Geometry: final body of the model. Coordinates: model frame, mm. Face numbers are marked on the shaded views. Round coordinates to 2 decimals unless told otherwise and drop trailing zeros. Loops run counter-clockwise (first coordinate to the right, second up) from the corner with the lowest first, then second, coordinate; pieces in that order, holes last. Notation, with made-up numbers: M 61,-37.5 L 100,-37.5 A21 ccw 100,-6.5 Z; hole C -16,67 d4. An arc over 180 degrees is marked long. Answer as a JSON object with one key per item and string values.
from build123d import *

# Parameters (mm, degrees)
SKETCH_1_W           = 300
SKETCH_1_H           = 30
EXTRUDE_1_DEPTH      = 20
EXTRUDE_2_DEPTH      = 28
EXTRUDE_2_DEPTH_BACK = 328
SKETCH_3_R           = 13.5
SKETCH_3_R_2         = 6
SKETCH_3_R_3         = 4
CUT_EXTRUDE_2_DEPTH  = 182.614977356
SKETCH_3_4_R         = 2.4
CUT_EXTRUDE_3_DEPTH  = 4.5
SKETCH_3_5_R         = 2.4
CUT_EXTRUDE_4_DEPTH  = 5


with BuildPart() as part:
    # Sketch 1 → Extrude 1 (new body)
    with BuildSketch(Plane.XY):
        with Locations((0, 15)):
            Rectangle(SKETCH_1_W, SKETCH_1_H)
    extrude(amount=EXTRUDE_1_DEPTH)

    # Sketch 2 → Extrude 2 (add, two sides: drawn at the far end of the back side and taken through both)
    with BuildSketch(Plane.ZY.offset(150).offset(-EXTRUDE_2_DEPTH_BACK)):
        with BuildLine():
            Line((0, 20), (0, 10))
            ThreePointArc((0, 10), (5, 15), (0, 20))
        make_face()
    extrude(amount=EXTRUDE_2_DEPTH + EXTRUDE_2_DEPTH_BACK)

    # Sketch 3 → Cut-Extrude 2 (cut, through all)
    # profile 1 of 3: a face of its own
    with BuildSketch(Plane(origin=(0, 0, 0), x_dir=(-1, 0, 0), z_dir=(0, 0, -1))):
        with Locations((0, 15)):
            Circle(SKETCH_3_R)
        with Locations((0, 15)):
            Circle(SKETCH_3_R_2, mode=Mode.SUBTRACT)
    # profile 2 of 3: a face of its own
    with BuildSketch(Plane(origin=(0, 0, 0), x_dir=(-1, 0, 0), z_dir=(0, 0, -1))):
        with Locations((0, 15)):
            Circle(SKETCH_3_R_2)
        with Locations((0, 15)):
            Circle(SKETCH_3_R_3, mode=Mode.SUBTRACT)
    # profile 3 of 3: a face of its own
    with BuildSketch(Plane(origin=(0, 0, 0), x_dir=(-1, 0, 0), z_dir=(0, 0, -1))):
        with Locations((0, 15)):
            Circle(SKETCH_3_R_3)
    extrude(amount=-CUT_EXTRUDE_2_DEPTH, mode=Mode.SUBTRACT)

    # Sketch 3_4 → Cut-Extrude 3 (cut)
    # profile 1 of 2: a face of its own
    with BuildSketch(Plane(origin=(0, 0, 0), x_dir=(-1, 0, 0), z_dir=(0, 0, -1))):
        with BuildLine():
            Line((25.573684211, 19.923075858), (4.689473684, 27.65933792))
            ThreePointArc((4.689473684, 27.65933792), (13.5, 15), (4.689473684, 2.34066208))
            Line((4.689473684, 2.34066208), (25.573684211, 10.076924142))
            ThreePointArc((25.573684211, 10.076924142), (29, 15), (25.573684211, 19.923075858))
        make_face()
        with Locations((23.75, 15)):
            Circle(SKETCH_3_4_R, mode=Mode.SUBTRACT)
    # profile 2 of 2: a face of its own
    with BuildSketch(Plane(origin=(0, 0, 0), x_dir=(-1, 0, 0), z_dir=(0, 0, -1))):
        with BuildLine():
            ThreePointArc((-4.689473684, 2.34066208), (-13.5, 15), (-4.689473684, 27.65933792))
            Line((-4.689473684, 27.65933792), (-25.573684211, 19.923075858))
            ThreePointArc((-25.573684211, 19.923075858), (-29, 15), (-25.573684211, 10.076924142))
            Line((-25.573684211, 10.076924142), (-4.689473684, 2.34066208))
        make_face()
        with Locations((-23.75, 15)):
            Circle(SKETCH_3_4_R, mode=Mode.SUBTRACT)
    extrude(amount=-CUT_EXTRUDE_3_DEPTH, mode=Mode.SUBTRACT)

    # Sketch 3_5 → Cut-Extrude 4 (cut)
    with BuildSketch(Plane(origin=(0, 0, 0), x_dir=(-1, 0, 0), z_dir=(0, 0, -1))):
        with Locations((-23.75, 15)):
            Circle(SKETCH_3_5_R)
        with Locations((23.75, 15)):
            Circle(SKETCH_3_5_R)
    extrude(amount=-CUT_EXTRUDE_4_DEPTH, mode=Mode.SUBTRACT)


solid = part.part
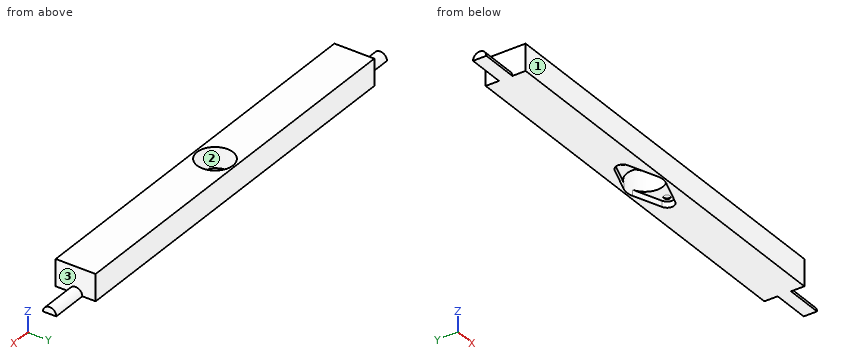
1) Pull-direction query (X, two-part tool) for the marked faces 1, 2 and 3; classes: +X half, -X half, draft (parallel to the pull), parting line (faces both ways), or undercut.
Results:
{"face 1": "draft", "face 2": "undercut", "face 3": "+X half"}
2) Ray query, line 1 (X direction, y = 14.25, z = 6.75); line 2 (Y direction, x = -23.75, z = 4.8); line 3 (Y direction, x = 0, z = 5.5). Return the intervals inside material, ascending.
Results:
{"line 1": "-150 to -13.48, 13.48 to 150", "line 2": "0 to 12.6, 17.4 to 30", "line 3": "0 to 1.5, 28.5 to 30"}
3) Section query B-B (z = 12.5). Return the cut outline in (x, y), and give its area (3 significant figures).
Results:
{"outline": "M -150,0 L 150,0 L 150,30 L -150,30 Z; hole C 0,15 d27", "area": "8,430 mm2"}
4) Section query C-C (x = -154). Return the cut outline in (y, z).
Results:
{"outline": "M 10,0 L 20,0 A5 ccw Z"}
5) Pin query (flat end, axial travel): P1, Ø7.5, axis at x = 18.5, y = 15.5, coming from the -Z side; P2, Ø2, axis at y = 11, z = 10.5, coming from the -X side. Return the tip coordinate at first contact, or that it passes through.
Results:
{"P1": "z = 4.5", "P2": "x = -150"}
6) Section query A-A (x = 0). Return the cut outline in (y, z).
Results:
{"outline": "M 0,0 L 1.5,0 L 1.5,20 L 0,20 Z; M 28.5,0 L 30,0 L 30,20 L 28.5,20 Z"}
